Could you check a few things on this drawing? It's one solid part, dimensions in mm from its lowest x, y, z. A direction names the side the tool comes from. Round coordinates to 2 decimals unless told otherwise and drop trailing zeros. Write each loop counter-clockwise with the first axis right and the second up, starting at its lowest first coordinate (ties: lowest second). Pieces come first, ordered by that corner, then holes. Notation, with made-up numbers: (88.25, 49.5) -> (117.25, 49.5) arc R27 ccw to (117.25, 76.5) -> close; hole circle Ø6 at (45.5, 20). An arc over 180 degrees is marked (long way). Put each result on its own line as item: value. Start each with the question number.
1) Which directions (+Z, -Z, +X, -X, +Y, -Y) give clear straight access to the entire face, cutting with the end or side of a thin tool? Please do the marked faces 1, 2 and 3.
2) I want a section at C-C, the plane y = 91.5. List the corners of the cut face in (x, z) for me.
3) I want a section at B-B, the plane z = 5.5. List the corners of the cut face in (x, y) for me.
4) If I drill on line 1 along Y through (x, z) = (11.5, 13); line 2 along Z through (x, y) = (7.25, 88); line 3 along X through (y, z) = (132, 10), over which ranges is the centre line in solid material (lowest first)? Write a range as [from, to].
5) We'd pull the mould along Y, two halves only. Please class the marked faces 4, 5 and 6: released by +Y, released by -Y, zero draft, split by the parting line, or undercut.
6) Will these pins go through, and if not, where does the flat tip stop? P1, Ø7.5, axis at y = 96, z = 3, coming from the -X side; P2, Ø5, axis at y = 95, z = 4.5, coming from the +X side; P3, Ø4, axis at x = 9.5, y = 42.5, coming from the +Z side.
7) I want a section at A-A, the plane x = 6.75. List the corners of the cut face in (y, z) for me.
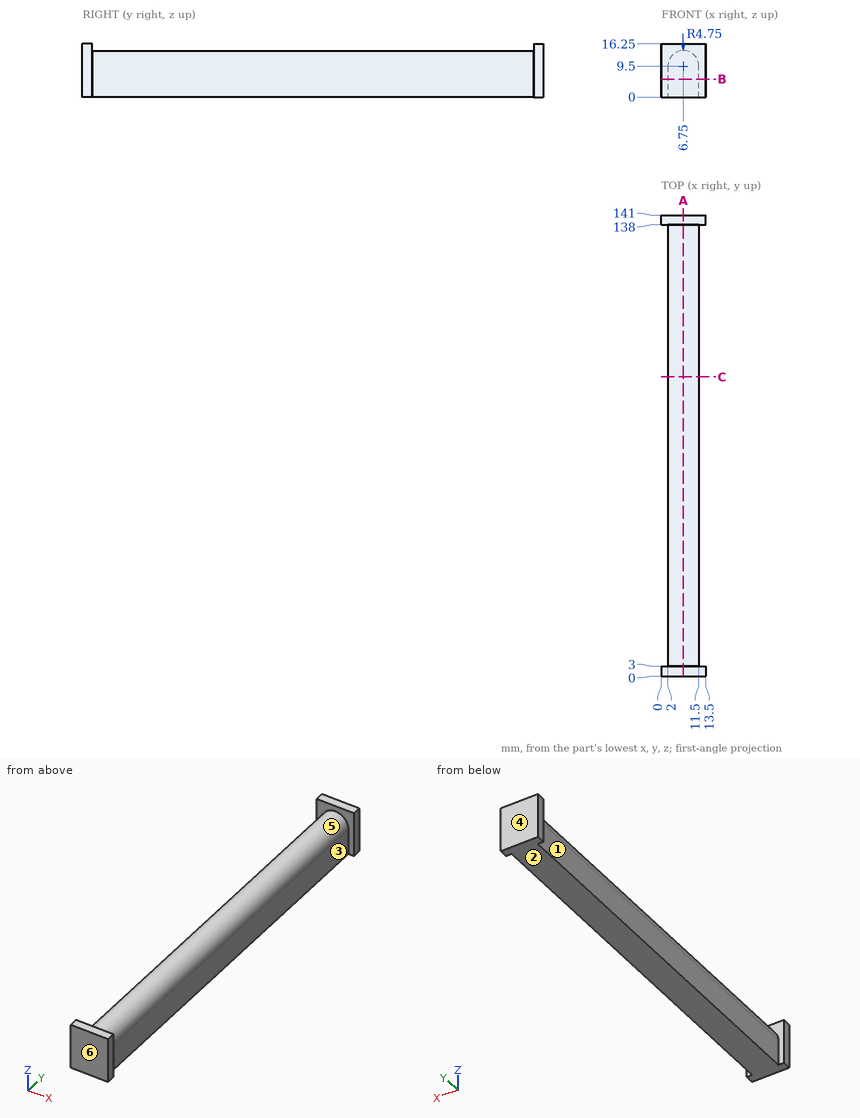
Findings:
1. face 1: +Z, -Z, -X
1. face 2: -Z, +X, -X, +Y, -Y
1. face 3: +Z, -Z, +X
2. outline: (2, 0) -> (11.5, 0) -> (11.5, 9.5) arc R4.75 ccw to (2, 9.5) -> close
3. outline: (0, 0) -> (13.5, 0) -> (13.5, 3) -> (11.5, 3) -> (11.5, 138) -> (13.5, 138) -> (13.5, 141) -> (0, 141) -> (0, 138) -> (2, 138) -> (2, 3) -> (0, 3) -> close
4. line 1: y = [0, 3], [138, 141]
4. line 2: z = [0, 14.22]
4. line 3: x = [2.03, 11.47]
5. face 4: released by +Y
5. face 5: undercut
5. face 6: released by -Y
6. P1: stops at x = 2
6. P2: stops at x = 11.5
6. P3: stops at z = 14.19
7. outline: (0, 0) -> (141, 0) -> (141, 16.25) -> (138, 16.25) -> (138, 14.25) -> (3, 14.25) -> (3, 16.25) -> (0, 16.25) -> close
